```python
from build123d import *
from OCP.BRepFilletAPI import BRepFilletAPI_MakeChamfer

# Parameters (mm, degrees)
CROQUIS2_W              = 421.86
CROQUIS2_H              = 289
SALIENTE_EXTRUIR1_DEPTH = 2.8
CROQUIS3_W              = 20
CROQUIS3_H              = 41
CORTAR_EXTRUIR1_DEPTH   = 2.8
SALIENTE_EXTRUIR2_DEPTH = 38
CORTAR_EXTRUIR2_DEPTH   = 415.044477804
CORTAR_EXTRUIR3_DEPTH   = 405.741435487
CROQUIS7_W              = 16.492420957
CROQUIS7_H              = 10.17289517
SALIENTE_EXTRUIR3_DEPTH = 6.06
CHAFL_N1_SIZE           = 6
CHAFL_N1_SIZE2          = 3.5
CROQUIS9_R              = 1.995453572
SALIENTE_EXTRUIR4_DEPTH = 8
CROQUIS10_W             = 18.263552833
CROQUIS10_H             = 19
SALIENTE_EXTRUIR5_DEPTH = 18
CORTAR_EXTRUIR4_DEPTH   = 410.374118869
SALIENTE_EXTRUIR6_DEPTH = 1
CROQUIS13_R             = 3
SALIENTE_EXTRUIR7_DEPTH = 20
CROQUIS18_R             = 1.55
CORTAR_EXTRUIR5_DEPTH   = 10


with BuildPart() as part:
    # Croquis2 → Saliente-Extruir1 (new body)
    with BuildSketch(Plane(origin=(0, 0, 0), x_dir=(1, 0, 0), z_dir=(0, 1, 0))):
        Rectangle(CROQUIS2_W, CROQUIS2_H)
    extrude(amount=SALIENTE_EXTRUIR1_DEPTH)

    # Croquis3 → Cortar-Extruir1 (cut)
    with BuildSketch(Plane(origin=(0, 2.8, 0), x_dir=(1, 0, 0), z_dir=(0, 1, 0))):
        with Locations((200.93, -124)):
            Rectangle(CROQUIS3_W, CROQUIS3_H)
        with Locations((200.93, 124)):
            Rectangle(CROQUIS3_W, CROQUIS3_H)
    extrude(amount=-CORTAR_EXTRUIR1_DEPTH, mode=Mode.SUBTRACT)

    # Croquis4 → Saliente-Extruir2 (add)
    with BuildSketch(Plane(origin=(0, 2.8, 0), x_dir=(1, 0, 0), z_dir=(0, 1, 0))):
        Polygon((174.93, 139.5), (99.93, 139.5), (99.93, 89.5), (99.93, 74.5), (164.93, 74.5), (164.93, 89.5), (174.93, 89.5), align=None)
    extrude(amount=SALIENTE_EXTRUIR2_DEPTH)

    # Croquis5 → Cortar-Extruir2 (cut, through all)
    with BuildSketch(Plane(origin=(174.93, 0, 0), x_dir=(0, 0, -1), z_dir=(1, 0, 0))):
        Polygon((89.5, 35.8), (101.5, 40.8), (89.5, 40.8), align=None)
    extrude(amount=-CORTAR_EXTRUIR2_DEPTH, mode=Mode.SUBTRACT)

    # Croquis6 → Cortar-Extruir3 (cut, through all)
    with BuildSketch(Plane(origin=(164.93, 0, 0), x_dir=(0, 0, -1), z_dir=(1, 0, 0))):
        Polygon((74.5, 35.8), (74.5, 20.8), (89.5, 35.8), (89.5, 40.8), (74.5, 40.8), align=None)
    extrude(amount=-CORTAR_EXTRUIR3_DEPTH, mode=Mode.SUBTRACT)

    # Croquis7 → Saliente-Extruir3 (add)
    with BuildSketch(Plane(origin=(0, 40.8, 0), x_dir=(1, 0, 0), z_dir=(0, 1, 0))):
        with Locations((152.683789521, 109.586447585)):
            Rectangle(CROQUIS7_W, CROQUIS7_H)
    extrude(amount=SALIENTE_EXTRUIR3_DEPTH)

    # Chaflán1: one chamfer whose edges measure the first distance from different faces: ONE call of the kernel's chamfer builder (chamfer() names one face for all edges)
    chafl_n1_edges_1 = [part.edges().sort_by_distance(p)[0] for p in [
        (160.93, 46.86, -109.586447585),
    ]]
    chafl_n1_side_1 = [part.faces().sort_by_distance(p)[0] for p in [
        (160.93, 43.83, -109.586447585),
    ]]
    chafl_n1_edges_2 = [part.edges().sort_by_distance(p)[0] for p in [
        (144.437579043, 46.86, -109.586447585),
    ]]
    chafl_n1_side_2 = [part.faces().sort_by_distance(p)[0] for p in [
        (144.437579043, 43.83, -109.586447585),
    ]]
    chafl_n1 = BRepFilletAPI_MakeChamfer(part.part.solid().wrapped)
    for e in chafl_n1_edges_1:
        chafl_n1.Add(CHAFL_N1_SIZE, CHAFL_N1_SIZE2, e.wrapped, chafl_n1_side_1[0].wrapped)  # the first distance lies on this face
    for e in chafl_n1_edges_2:
        chafl_n1.Add(CHAFL_N1_SIZE, CHAFL_N1_SIZE2, e.wrapped, chafl_n1_side_2[0].wrapped)  # the first distance lies on this face
    add(Compound.cast(chafl_n1.Shape()), mode=Mode.REPLACE)

    # Croquis9 → Saliente-Extruir4 (add)
    with BuildSketch(Plane(origin=(0, 46.86, 0), x_dir=(1, 0, 0), z_dir=(0, 1, 0))):
        with Locations(Location((152.683789521, 109.586447585, 0), (0, 0, 270))):
            Circle(CROQUIS9_R)
    extrude(amount=SALIENTE_EXTRUIR4_DEPTH)

    # Croquis10 → Saliente-Extruir5 (add)
    with BuildSketch(Plane(origin=(0, 0, -139.5), x_dir=(-1, 0, 0), z_dir=(0, 0, -1))):
        with Locations((-153.798223584, 31.3)):
            Rectangle(CROQUIS10_W, CROQUIS10_H)
    extrude(amount=SALIENTE_EXTRUIR5_DEPTH)

    # Croquis11 → Cortar-Extruir4 (cut, through all)
    with BuildSketch(Plane(origin=(162.93, 0, 0), x_dir=(0, 0, -1), z_dir=(1, 0, 0))):
        Polygon((157.5, 38.8), (143.909536757, 21.8), (157.5, 21.8), align=None)
    extrude(amount=-CORTAR_EXTRUIR4_DEPTH, mode=Mode.SUBTRACT)

    # Croquis12 → Saliente-Extruir6 (add)
    with BuildSketch(Plane(origin=(0, 40.8, 0), x_dir=(1, 0, 0), z_dir=(0, 1, 0))):
        with BuildLine():
            ThreePointArc((160.298223583, 148.5), (156.263827828, 154.514216134), (149.168747981, 153.062669794))
            Line((149.168747981, 153.062669794), (158.427699186, 143.937330206))
            ThreePointArc((158.427699186, 143.937330206), (159.812439717, 146.034395755), (160.298223583, 148.5))
        make_face()
        with BuildLine():
            Line((158.427699186, 143.937330206), (149.168747981, 153.062669794))
            ThreePointArc((149.168747981, 153.062669794), (149.23555379, 143.870524398), (158.427699186, 143.937330206))
        make_face()
    extrude(amount=SALIENTE_EXTRUIR6_DEPTH)

    # Croquis13 → Saliente-Extruir7 (add)
    with BuildSketch(Plane(origin=(0, 41.8, 0), x_dir=(1, 0, 0), z_dir=(0, 1, 0))):
        with Locations(Location((153.798223583, 148.5, 0), (0, 0, 270))):
            Circle(CROQUIS13_R)
    extrude(amount=SALIENTE_EXTRUIR7_DEPTH)

    # Croquis18 → Cortar-Extruir5 (cut)
    with BuildSketch(Plane(origin=(0, 2.8, 0), x_dir=(1, 0, 0), z_dir=(0, 1, 0))):
        with Locations(Location((-177.78113513, 112.490742036, 0), (0, 0, 270))):
            Circle(CROQUIS18_R)
        with Locations(Location((-177.78113513, 140.790742036, 0), (0, 0, 270))):
            Circle(CROQUIS18_R)
        with Locations(Location((-202.78113513, 126.640742036, 0), (0, 0, 270))):
            Circle(CROQUIS18_R)
    extrude(amount=-CORTAR_EXTRUIR5_DEPTH, mode=Mode.SUBTRACT)


solid = part.part
```
For this review, take the finished solid that the model builds, in its own axes (mm). A direction names the side the tool comes from. Round coordinates to 2 decimals unless told otherwise and drop trailing zeros. Order: outer loops, then holes, each group sorted by start corner. A loop starts at its lowest first (then second) coordinate and runs counter-clockwise, first axis right, second up.
Q1. We need section A-A, the plane x = -169. Give the boundary of the cut face in (y, z).
Findings below:
outline: (0, -144.5) - (2.8, -144.5) - (2.8, 144.5) - (0, 144.5) - close
Q2. Mouldability with a two-part tool opening along Z and no side actions: class faces 1 (the flat face through (-3, 0, -2)), 2 (the flat face through (170, 19, -89.5)), 3 (the flat face through (150.5, 46.86, -109.7)) as pulls with the +Z half, pulls with the -Z half, needs draft (parallel to the pull), parting line crosses it, or undercut.
Findings below:
face 1: needs draft
face 2: pulls with the +Z half
face 3: undercut
Q3. We need section B-B, the plane y = 28.5. Give the boundary of the cut face in (x, z), plus the area to 3 significant figures.
Findings below:
outline: (99.93, -139.5) - (144.67, -139.5) - (144.67, -149.27) - (162.93, -149.27) - (162.93, -139.5) - (174.93, -139.5) - (174.93, -89.5) - (164.93, -89.5) - (164.93, -82.2) - (99.93, -82.2) - close
area: 4,400 mm2
Q4. Wall thickness on line 1 (Y direction, x = -29.5, z = -40); line 2 (X direction, y = 11, z = -93.5); line 3 (Z direction, x = 158, y = 4.5): over which ranges is each line inside the solid? List them lowest first.
Findings below:
line 1: y = 0 to 2.8
line 2: x = 99.93 to 174.93
line 3: z = -139.5 to -74.5
Q5. Machinability: for faces 4 (the flat face through (174.93, 22, -114)), 5 (the flat face through (144.666, 33, -146)), 6 (the flat face through (99.93, 22, -107)), 7 (the flat face through (157, 41.8, -147)), which of the approach directions +Z, -Z, +X, -X, +Y, -Y give a long, thin tool a straight path to every point of the face, cutting with its end or side? Answer none if there is none.
Findings below:
face 4: +Z, -Z, +X, +Y
face 5: -Z, -X, +Y
face 6: +Z, -Z, -X, +Y
face 7: +Y
Q6. Insertion check: P1, Ø8, axis at x = -60.5, z = -57.5, coming from the +Y side; P2, Ø17, axis at x = 148.5, z = -133, coming from the +Y side; P3, Ø1.8, axis at x = 151, y = 45, coming from the -Z side. Each pin has a flat end and moves straight along its axis. Give the tip position at first contact, or say it passes through.
Findings below:
P1: stops at y = 2.8
P2: stops at y = 40.8
P3: stops at z = -150.82
